from build123d import *

# Parameters (mm, degrees)
F0_W     = 40
F0_H     = 40
F0_R     = 0.3
F1_DEPTH = 2.4


# Not quite as in the source:
# - a fillet or chamfer that OpenCascade refuses, or shapes differently, is made with other operations: its cross-section is extruded or revolved along the edge and cut away or added


with BuildPart() as f1:
    # F0 (on Top) → F1 (new body)
    with BuildSketch(Plane.XY):
        Rectangle(F0_W, F0_H)
        with Locations((-12, -12)):
            Circle(F0_R, mode=Mode.SUBTRACT)
        with Locations((12, -12)):
            Circle(F0_R, mode=Mode.SUBTRACT)
        with Locations((-12, 12)):
            Circle(F0_R, mode=Mode.SUBTRACT)
        with Locations((12, 12)):
            Circle(F0_R, mode=Mode.SUBTRACT)
    extrude(amount=F1_DEPTH)

    # F2: chamfer of 2.5 on 4 edges, made by hand

    # F2_s1 → F2_t2 (revolve, cut)
    with BuildSketch(Plane.XZ.offset(-12)):
        Polygon((-11.7, -0.1), (-9.2, 2.4), (-11.7, 2.4), align=None)
    revolve(axis=Axis((-12, 12, 2.4), (0, 0, 1)), mode=Mode.SUBTRACT)

    # F2_s3 → F2_t4 (revolve, cut)
    with BuildSketch(Plane.XZ.offset(-12)):
        Polygon((12.3, -0.1), (14.8, 2.4), (12.3, 2.4), align=None)
    revolve(axis=Axis((12, 12, 2.4), (0, 0, 1)), mode=Mode.SUBTRACT)

    # F2_s5 → F2_t6 (revolve, cut)
    with BuildSketch(Plane.XZ.offset(12)):
        Polygon((12.3, -0.1), (14.8, 2.4), (12.3, 2.4), align=None)
    revolve(axis=Axis((12, -12, 2.4), (0, 0, 1)), mode=Mode.SUBTRACT)

    # F2_s7 → F2_t8 (revolve, cut)
    with BuildSketch(Plane.XZ.offset(12)):
        Polygon((-11.7, -0.1), (-9.2, 2.4), (-11.7, 2.4), align=None)
    revolve(axis=Axis((-12, -12, 2.4), (0, 0, 1)), mode=Mode.SUBTRACT)


solid = f1.part
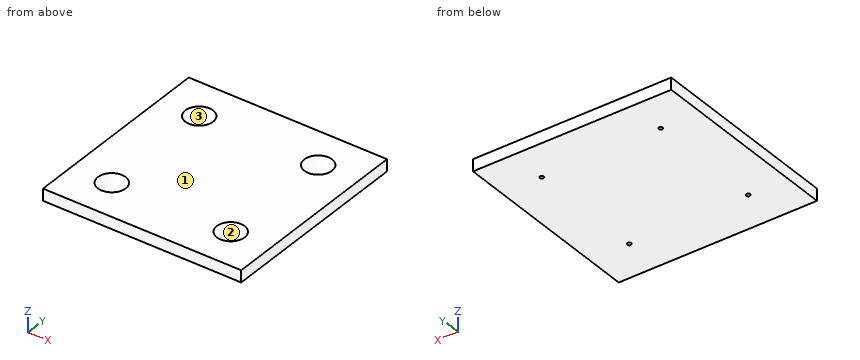
Can you work these out from the model? Positions are in its coordinate system, mm. Face numbers are marked on the shaded views. Coordinates: 2 decimals unless noted, no trailing zeros. Loops run counter-clockwise (first coordinate to the right, second up) from the corner with the lowest first, then second, coordinate; pieces in that order, holes last. Notation, with made-up numbers: M -9,26.25 L 17,26.25 A11 ccw 17,33.25 Z; hole C 7.5,82 d6. An arc over 180 degrees is marked long. Answer as CSV lines item,"result". Start each with the question number.
1. Suppose I cut it at A-A, the plane y = 12. List the corners of the cut face in (x, z) for me.
2. Thinking about a two-plate mould opening in X: for the marked faces 1, 2 and 3, which applies, +X half, -X half, draft (parallel to the pull), parting line (faces both ways), or undercut?
3. Suppose I cut it at B-B, the plane z = 1.75. List the corners of the cut face in (x, y) for me.
4. If I drill on probe 1 along Y at (x, z) = (12, 0.55); probe 2 along X at (y, z) = (12, 1.45); probe 3 along Y at (x, z) = (11.5, 0.35), over which ranges is the centre line in solid material (lowest first)? Write a range as [from, to].
Output:
1,outline,"M -20,0 L -12.4,0 L -14.8,2.4 L -20,2.4 Z; M -11.6,0 L 11.6,0 L 9.2,2.4 L -9.2,2.4 Z; M 12.4,0 L 20,0 L 20,2.4 L 14.8,2.4 Z"
2,face 1,"draft"
2,face 2,"undercut"
2,face 3,"undercut"
3,outline,"M -20,-20 L 20,-20 L 20,20 L -20,20 Z; hole C -12,-12 d4.3; hole C -12,12 d4.3; hole C 12,-12 d4.3; hole C 12,12 d4.3"
4,probe 1,"y = [-20, -12.95], [-11.05, 11.05], [12.95, 20]"
4,probe 2,"x = [-20, -13.85], [-10.15, 10.15], [13.85, 20]"
4,probe 3,"y = [-20, -12.56], [-11.44, 11.44], [12.56, 20]"
